from build123d import *

# Parameters (mm, degrees)
F0_R     = 88.786402
F1_DEPTH = 31.552652
F2_R     = 28.067948
F3_DEPTH = 295.643002
F4_SIZE  = 5.08
F5_SIZE  = 5.08


with BuildPart() as f1:
    # F0 (on Right) → F1 (new body)
    with BuildSketch(Plane.YZ):
        Circle(F0_R)
    extrude(amount=F1_DEPTH)

    # F2 (on face) → F3 (join)
    with BuildSketch(Plane(origin=(0, 0, 0), x_dir=(0, -1, 0), z_dir=(-1, 0, 0))):
        Circle(F2_R)
    extrude(amount=F3_DEPTH)

    # F4
    f4_edges = [f1.edges().sort_by_distance(p)[0] for p in [
        (-147.821501, -28.067948, 0),
        (0, 28.067948, 0),
        (-295.643002, 28.067948, 0),
    ]]
    chamfer(f4_edges, length=F4_SIZE)

    # F5
    f5_edges = [f1.edges().sort_by_distance(p)[0] for p in [
        (31.552652, -88.786402, 0),
        (0, -88.786402, 0),
    ]]
    chamfer(f5_edges, length=F5_SIZE)


solid = f1.part
Here's how the part is built. I have some questions about the finished solid (model axes, mm). A direction names the side the tool comes from. Give positions to 0.01 mm unless a question says otherwise; leave off trailing zeros. Order: outer loops, then holes, each group sorted by start corner. A loop starts at its lowest first (then second) coordinate and runs counter-clockwise, first axis right, second up. Notation, with made-up numbers: M 15,-4.75 L 73,-4.75 A24 ccw 73,21.25 Z; hole C 70.25,55 d3. An arc over 180 degrees is marked long. Answer as a JSON object with one key per item and string values. Group by question number.
1) Please list where these lines run through material, in increasing order: L1, parallel to X at y = -50.5, z = -42.5; L2, parallel to Y at x = -273, z = 17.5; L3, parallel to Z at x = -25, y = -10.5. Write a range as [from, to].
2) I'm going to push flat-ended pins straight in: pin 1 Ø10 at (y, z) = (30, -65.5) entering from -X; pin 2 Ø2 at (x, z) = (-197.5, 22.5) entering from -Y; pin 3 Ø4 at (x, y) = (-48.5, 2) entering from +Z. Where does each tip first touch, or does it pass through?
3) Suppose I cut it at C-C, the plane x = -60.5. Write out the boundary of the cut face in (y, z).
4) Suppose I cut it at A-A, the plane z = 0. Write out the boundary of the cut face in (x, y), plus the area to 3 significant figures.
5) On a 3-axis mill with a long thin cutter (end or side, diameter ignored), from which of +Z, -Z, +X, -X, +Y, -Y can I reach the whole of each face in a straight line? I mean faces 1 (the flat face through (0, 36, 1)), 2 (the flat face through (31.553, -1, 1)). Say none if no direction works.
Results found:
{
 "1": {"L1": "[0, 31.55]", "L2": "[-21.94, 21.94]", "L3": "[-26.03, 26.03]"},
 "2": {"pin 1": "x = 0", "pin 2": "y = -18.04", "pin 3": "z = 28.07"},
 "3": {"outline": "C 0,0 d56.14"},
 "4": {"outline": "M -295.64,-22.99 L -290.56,-28.07 L -5.08,-28.07 L 0,-33.15 L 0,-83.71 L 5.08,-88.79 L 26.47,-88.79 L 31.55,-83.71 L 31.55,83.71 L 26.47,88.79 L 5.08,88.79 L 0,83.71 L 0,33.15 L -5.08,28.07 L -290.56,28.07 L -295.64,22.99 Z", "area": "22,100 mm²"},
 "5": {"face 1": "-X", "face 2": "+Z, -Z, +X, +Y, -Y"}
}
